```python
from build123d import *

# Parameters (mm, degrees)
BLANKSKE_W          = 48.375
BLANKSKE_H          = 7
BLANK_DEPTH         = 5
TOOTHCUTSIM_DEPTH   = 50.133905045
TEETHCUTS_COUNT     = 18
TEETHCUTS_PITCH     = 2.827433385
SKETCH7_W           = 6.878661204
SKETCH7_H           = 4.975
BOSS_EXTRUDE5_DEPTH = 48.375
SKETCH8_R           = 2.6
BOSS_EXTRUDE6_DEPTH = 32
SKETCH10_W          = 3
SKETCH10_H          = 2.75
BOSS_EXTRUDE8_DEPTH = 48.375
SKETCH11_W          = 3
SKETCH11_H          = 3
BOSS_EXTRUDE9_DEPTH = 6.15
SKETCH12_W          = 3
SKETCH12_H          = 2
CUT_EXTRUDE1_DEPTH  = 0.5


with BuildPart() as part:
    # BlankSke → Blank (new body)
    with BuildSketch(Plane.XY):
        with Locations((24.1875, 3.5)):
            Rectangle(BLANKSKE_W, BLANKSKE_H)
    extrude(amount=-BLANK_DEPTH)

    # TooCutSkeSim → ToothCutSim (cut, through all)
    with BuildSketch(Plane.XY):
        Polygon((0.399391833, 4.975), (-0.399391833, 4.975), (-1.145676401, 7.0254), (1.145676401, 7.0254), align=None)
    toothcutsim = extrude(amount=-TOOTHCUTSIM_DEPTH, mode=Mode.SUBTRACT)

    # TeethCuts: ToothCutSim ×18
    with Locations(*[(i * TEETHCUTS_PITCH, 0, 0) for i in range(1, TEETHCUTS_COUNT)]):
        add(toothcutsim, mode=Mode.SUBTRACT)

    # Sketch7 → Boss-Extrude5 (add)
    with BuildSketch(Plane(origin=(48.375, 0, 0), x_dir=(0, 0, -1), z_dir=(1, 0, 0))):
        with Locations((-3.439330602, 2.4875)):
            Rectangle(SKETCH7_W, SKETCH7_H)
    extrude(amount=-BOSS_EXTRUDE5_DEPTH)

    # Sketch8 → Boss-Extrude6 (add)
    with BuildSketch(Plane(origin=(48.375, 0, 0), x_dir=(0, 0, -1), z_dir=(1, 0, 0))):
        with Locations(Location((-4.278661804, 2.489267286, 0), (0, 0, 180))):
            Circle(SKETCH8_R)
    extrude(amount=BOSS_EXTRUDE6_DEPTH)

    # Sketch10 → Boss-Extrude8 (add)
    with BuildSketch(Plane.ZY):
        with Locations((5.378661204, 6.35)):
            Rectangle(SKETCH10_W, SKETCH10_H)
    boss_extrude8 = extrude(amount=-BOSS_EXTRUDE8_DEPTH)

    # Mirror6: Boss-Extrude8 across plane
    add(boss_extrude8.mirror(Plane.ZX.offset(2.4875)))

    # Sketch11 → Boss-Extrude9 (add)
    with BuildSketch(Plane.XZ.offset(2.75)):
        with Locations((1.5, 5.378661204)):
            Rectangle(SKETCH11_W, SKETCH11_H)
    boss_extrude9 = extrude(amount=BOSS_EXTRUDE9_DEPTH)

    # Mirror7: Boss-Extrude9 across plane
    add(boss_extrude9.mirror(Plane.ZX.offset(2.4875)))

    # Sketch12 → Cut-Extrude1 (cut)
    with BuildSketch(Plane.ZY):
        with Locations((5.378661204, -6.9)):
            Rectangle(SKETCH12_W, SKETCH12_H)
    cut_extrude1 = extrude(amount=-CUT_EXTRUDE1_DEPTH, mode=Mode.SUBTRACT)

    # Mirror8: Cut-Extrude1 across plane
    add(cut_extrude1.mirror(Plane.ZX.offset(2.4875)), mode=Mode.SUBTRACT)


solid = part.part
```
Can you work these out from the model? Positions are in its coordinate system, mm. A direction names the side the tool comes from. Coordinates: 2 decimals unless noted, no trailing zeros. Loops run counter-clockwise (first coordinate to the right, second up) from the corner with the lowest first, then second, coordinate; pieces in that order, holes last.
Item 1: Suppose I cut it at A-A (y = 8.5). Please give me the cut outline in (x, z), then the cut area to 3 significant figures.
Answers below:
outline: (0, 3.88) - (3, 3.88) - (3, 6.88) - (0, 6.88) - close
area: 9.00 mm2
Item 2: If we mould it in two halves opening along Y, with no side actions, what happens to faces 4 (the face through (3, 11, 5)), 5 (the face through (19.2, 4.975, 0.5))? For each: released by +Y, released by -Y, zero draft, split by the parting line, or undercut.
Answers below:
face 4: zero draft
face 5: released by +Y
Item 3: Which directions (+Z, -Z, +X, -X, +Y, -Y) give clear straight access to the entire face, cutting with the end or side of a thin tool? Please do faces 1 (the face through (27, 6, 0)), 2 (the face through (80.375, 2, 4)), 3 (the face through (2.065, 5.973, -2.465)).
Answers below:
face 1: +X, -X, +Y
face 2: +Z, -Z, +X, +Y, -Y
face 3: -Z, +Y
Item 4: Please list where these lines run through material, in increasing order: L1, parallel to Y at x = 43, z = 6.25 (3 decimals); L2, parallel to Y at x = 23, z = 2.5 (3 decimals); L3, parallel to Z at x = 60, y = 2.5.
Answers below:
L1: y = -2.75 to 7.725
L2: y = 0 to 4.975
L3: z = 1.68 to 6.88
Item 5: Suppose I cut it at C-C (x = 69). Please give me the cut outline in (y, z), then the cut area to 3 significant figures.
Answers below:
outline: circle Ø5.2 at (2.49, 4.28)
area: 21.2 mm2
Item 6: I'm going to push flat-ended pins straight in: pin 1 (1.5 mm diameter, centred on x = 69.5, z = 3.5, fed in from +Y); pin 2 (0.6 mm diameter, centred on x = 1.5, z = -2, fed in from +Y); pin 3 (5 mm diameter, centred on x = 69, z = -0.5, fed in from +Y); pin 4 (6 mm diameter, centred on y = 11, z = 0.5, fed in from -X). Where does each tip first touch, or does it pass through?
Answers below:
pin 1: stops at y = 5.09
pin 2: stops at y = 7
pin 3: stops at y = 3.74
pin 4: passes through
Item 7: Suppose I cut it at B-B (z = 5.75). Please give me the cut outline in (x, y) (3 decimals).
Answers below:
outline: (0, -8.9) - (3, -8.9) - (3, -2.75) - (48.375, -2.75) - (48.375, 0.346) - (80.375, 0.346) - (80.375, 4.633) - (48.375, 4.633) - (48.375, 7.725) - (3, 7.725) - (3, 13.875) - (0, 13.875) - (0, 12.875) - (0.5, 12.875) - (0.5, 10.875) - (0, 10.875) - (0, -5.9) - (0.5, -5.9) - (0.5, -7.9) - (0, -7.9) - close
